```python
from build123d import *

# Parameters (mm, degrees)
PIN_DRAWING_W       = 0.636
PIN_DRAWING_H       = 0.636
BOSS_EXTRUDE1_DEPTH = 2.54


with BuildPart() as part:
    # pin_drawing → Boss-Extrude1 (new body)
    with BuildSketch(Plane.XY):
        Polygon((-0.014377737, 2.079116284), (-0.014377737, 0.25314904), (0.339175653, -0.107330326), (-0.014377737, -0.460883716), (-0.014377737, -2.28685096), (0.339175653, -2.647330326), (2.164719162, -2.647330326), (2.518272553, -2.293776935), (2.518272553, -0.46648), (2.164719162, -0.107330326), (2.518272553, 0.246223065), (2.518272553, 2.07352), (2.164719162, 2.432669674), (2.518272553, 2.786223065), (2.518272553, 4.61352), (2.164719162, 4.972669674), (2.518272553, 5.326223065), (2.518272553, 7.15352), (2.164719162, 7.512669674), (2.518272553, 7.866223065), (2.518272553, 9.69352), (2.164719162, 10.052669674), (2.518272553, 10.406223065), (2.518272553, 12.23352), (2.164719162, 12.592669674), (2.518272553, 12.946223065), (2.518272553, 14.77352), (2.164719162, 15.132669674), (2.518272553, 15.486223065), (2.518272553, 17.31352), (2.164719162, 17.672669674), (0.339175653, 17.672669674), (-0.014377737, 17.319116284), (-0.014377737, 15.49314904), (0.339175653, 15.132669674), (-0.014377737, 14.779116284), (-0.014377737, 12.95314904), (0.339175653, 12.592669674), (-0.014377737, 12.239116284), (-0.014377737, 10.41314904), (0.339175653, 10.052669674), (-0.014377737, 9.699116284), (-0.014377737, 7.87314904), (0.339175653, 7.512669674), (-0.014377737, 7.159116284), (-0.014377737, 5.33314904), (0.339175653, 4.972669674), (-0.014377737, 4.619116284), (-0.014377737, 2.79314904), (0.339175653, 2.432669674), align=None)
        with Locations((1.256122263, -1.357330326)):
            Rectangle(PIN_DRAWING_W, PIN_DRAWING_H, mode=Mode.SUBTRACT)
        with Locations((1.256122263, 1.182669674)):
            Rectangle(PIN_DRAWING_W, PIN_DRAWING_H, mode=Mode.SUBTRACT)
        with Locations((1.256122263, 3.722669674)):
            Rectangle(PIN_DRAWING_W, PIN_DRAWING_H, mode=Mode.SUBTRACT)
        with Locations((1.256122263, 6.262669674)):
            Rectangle(PIN_DRAWING_W, PIN_DRAWING_H, mode=Mode.SUBTRACT)
        with Locations((1.256122263, 8.802669674)):
            Rectangle(PIN_DRAWING_W, PIN_DRAWING_H, mode=Mode.SUBTRACT)
        with Locations((1.256122263, 11.342669674)):
            Rectangle(PIN_DRAWING_W, PIN_DRAWING_H, mode=Mode.SUBTRACT)
        with Locations((1.256122263, 13.882669674)):
            Rectangle(PIN_DRAWING_W, PIN_DRAWING_H, mode=Mode.SUBTRACT)
        with Locations((1.256122263, 16.422669674)):
            Rectangle(PIN_DRAWING_W, PIN_DRAWING_H, mode=Mode.SUBTRACT)
    extrude(amount=BOSS_EXTRUDE1_DEPTH)


solid = part.part
```
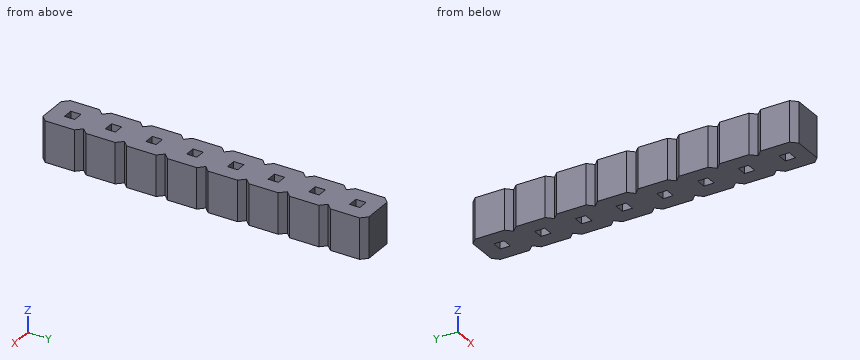
Verification items for the finished model (mm, model axes). Give positions to 0.01 mm unless a question says otherwise; leave off trailing zeros. Order: outer loops, then holes, each group sorted by start corner. A loop starts at its lowest first (then second) coordinate and runs counter-clockwise, first axis right, second up. Notation, with made-up numbers: M 85.5,45 L 139.5,45 A14 ccw 139.5,64 Z; hole C 3.5,67 d4. An arc over 180 degrees is marked long. Return JSON: item names as keys, results as strings. Group by question number.
1) Section check A-A on y = 1.25. Record the cut outline in (x, z), and give its area (3 significant figures).
2) Scan lines: line 1 (X direction, y = 3.5, z = 1.55); line 2 (X direction, y = 2.5, z = 2.05); line 3 (X direction, y = 15, z = 1.6). Record each from-to range of solid material in increasing order.
3) Section check B-B on x = 2.35. Give the number of separate pieces and of enclosed holes in the cut face, and give its area (3 significant figures).
Answer block:
{
 "1": {"outline": "M -0.01,0 L 0.94,0 L 0.94,2.54 L -0.01,2.54 Z; M 1.57,0 L 2.52,0 L 2.52,2.54 L 1.57,2.54 Z", "area": "4.82 mm^2"},
 "2": {"line 1": "x = -0.01 to 0.94, 1.57 to 2.52", "line 2": "x = 0.27 to 2.23", "line 3": "x = 0.21 to 2.3"},
 "3": {"separate pieces": "8", "enclosed holes": "0", "area": "44.0 mm^2"}
}
